Check sheet for the modelled part. Datum: model origin and axes. Units: mm. Face numbers are marked on the shaded views. Round coordinates to 2 decimals unless told otherwise and drop trailing zeros. Order: outer loops, then holes, each group sorted by start corner. A loop starts at its lowest first (then second) coordinate and runs counter-clockwise, first axis right, second up.
(1) Sectioned sample at D-D, the plane z = -78. Enter the section's corners in (x, y).
(2) Depth check by flat-ended pin: pin 1 (7.5 mm diameter, centred on x = 162, y = 28, fed in from +Z); pin 2 (4 mm diameter, centred on x = 153.5, z = -108.5, fed in from +Y); pin 3 (7.5 mm diameter, centred on x = 15, y = 18.5, fed in from -Z). Enter the tip coordinate at first touch or a pass-through.
(3) Thickness scan on probe 1 along Y at (x, z) = (172.05, -51); probe 2 along Y at (x, z) = (3.95, -42.5); probe 3 along X at (y, z) = (16, -122). Record the ranges inside material, lowest first.
(4) Mould release check, pull along Z, two halves, no side actions. Record for the marked faces 1 and 2: released by +Z, released by -Z, zero draft, split by the parting line, or undercut.
(5) Sectioned sample at B-B, the plane x = 72. Enter the section's corners in (y, z).
(6) Sectioned sample at C-C, the plane z = -117.5. Enter the section's corners in (x, y), and give its area (4 significant figures).
(7) Sectioned sample at A-A, the plane z = -157.5. Enter the section's corners in (x, y).
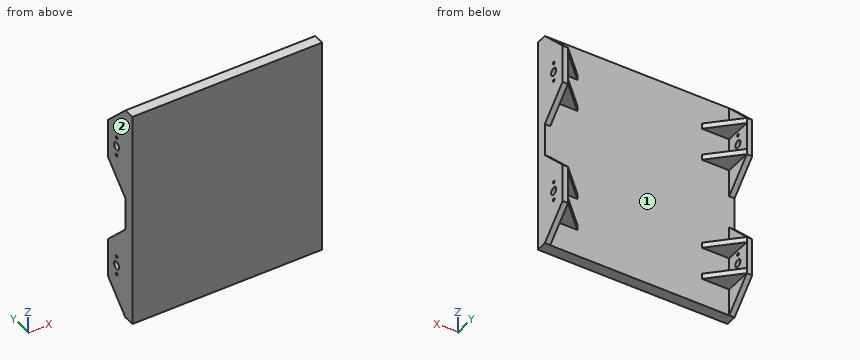
```python
from build123d import *

# Parameters (mm, degrees)
SKETCH1_W                = 175
SKETCH1_H                = 200
BOSS_EXTRUDE1_DEPTH      = 10
SKETCH3_W                = 5
SKETCH3_H                = 25
SKETCH3_W_2              = 25
SKETCH3_H_2              = 5
BOSS_EXTRUDE2_DEPTH      = 25
CHAMFER1_SIZE            = 25
SKETCH4_R                = 3.5
SKETCH4_R_2              = 1.25
CUT_EXTRUDE1_DEPTH       = 25
CHAMFER1_OF_MIRROR1_SIZE = 25


# Read off the part's stored shape, not the designer's step: Mirror2
with BuildPart() as part:
    # Sketch1 → Boss-Extrude1 (new body)
    with BuildSketch(Plane(origin=(0, 0, 0), x_dir=(1, 0, 0), z_dir=(0, 1, 0))):
        with Locations((87.5, 100)):
            Rectangle(SKETCH1_W, SKETCH1_H)
    extrude(amount=BOSS_EXTRUDE1_DEPTH)

    # Sketch3 → Boss-Extrude2 (add)
    with BuildSketch(Plane(origin=(0, 10, 0), x_dir=(1, 0, 0), z_dir=(0, 1, 0))):
        with Locations((2.5, 72.5)):
            Rectangle(SKETCH3_W, SKETCH3_H)
        Polygon((0, 60), (0, 25), (5, 25), (5, 30), (5, 55), (5, 60), align=None)
        with Locations((17.5, 57.5)):
            Rectangle(SKETCH3_W_2, SKETCH3_H_2)
        with Locations((17.5, 27.5)):
            Rectangle(SKETCH3_W_2, SKETCH3_H_2)
        with Locations((2.5, 12.5)):
            Rectangle(SKETCH3_W, SKETCH3_H)
    boss_extrude2 = extrude(amount=BOSS_EXTRUDE2_DEPTH)

    # Chamfer1
    chamfer1_edges = [part.edges().sort_by_distance(p)[0] for p in [
        (2.5, 35, -85),
        (30, 35, -57.5),
        (30, 35, -27.5),
        (2.5, 35, 0),
    ]]
    chamfer(chamfer1_edges, length=CHAMFER1_SIZE - 0.0001)  # a hair under: the kernel refuses the full size

    # Sketch4 → Cut-Extrude1 (cut)
    with BuildSketch(Plane(origin=(5, 0, 0), x_dir=(0, 0, -1), z_dir=(1, 0, 0))):
        with Locations((42.5, 22.5)):
            Circle(SKETCH4_R)
        with Locations((34, 22.5)):
            Circle(SKETCH4_R_2)
        with Locations((51, 22.5)):
            Circle(SKETCH4_R_2)
    cut_extrude1 = extrude(amount=-CUT_EXTRUDE1_DEPTH, mode=Mode.SUBTRACT)

    # Mirror1: Boss-Extrude2, Cut-Extrude1 across plane
    add(boss_extrude2.mirror(Plane(origin=(87.5, 0, 0), x_dir=(0, 0, 1), z_dir=(1, 0, 0))))
    add(cut_extrude1.mirror(Plane(origin=(87.5, 0, 0), x_dir=(0, 0, 1), z_dir=(1, 0, 0))), mode=Mode.SUBTRACT)

    # Chamfer1 of Mirror1
    chamfer1_of_mirror1_edges = [part.edges().sort_by_distance(p)[0] for p in [
        (172.5, 35, -85),
        (145, 35, -57.5),
        (145, 35, -27.5),
        (172.5, 35, 0),
    ]]
    chamfer(chamfer1_of_mirror1_edges, length=CHAMFER1_OF_MIRROR1_SIZE - 0.0001)  # a hair under: the kernel refuses the full size

    # Mirror2: part across plane


with BuildPart() as part_1:
    add(part.part)
    add(part.part.mirror(Plane.XY.offset(-100)))


solid = part_1.part
```
Derived:
1. outline: (0, 0) - (175, 0) - (175, 17) - (170, 17) - (170, 10) - (5, 10) - (5, 17) - (0, 17) - close
2. pin 1: stops at z = -25
2. pin 2: stops at y = 10
2. pin 3: stops at z = -175
3. probe 1: y = 0 to 21.25, 23.75 to 35
3. probe 2: y = 0 to 19, 26 to 35
3. probe 3: x = 0 to 5, 170 to 175
4. face 1: undercut
4. face 2: zero draft
5. outline: (0, -200) - (10, -200) - (10, 0) - (0, 0) - close
6. outline: (0, 0) - (175, 0) - (175, 12.5) - (170, 12.5) - (170, 10) - (5, 10) - (5, 12.5) - (0, 12.5) - close
6. area: 1,775 mm2
7. outline: (0, 0) - (175, 0) - (175, 19) - (170, 19) - (170, 10) - (5, 10) - (5, 19) - (0, 19) - close; (0, 26) - (5, 26) - (5, 35) - (0, 35) - close; (170, 26) - (175, 26) - (175, 35) - (170, 35) - close
